Autodesk Inventor part; units mm, degrees
ref_plane "YZ Plane" through (0, 0, 0) normal (1, 0, 0) x (0, 1, 0)
ref_plane "XZ Plane" through (0, 0, 0) normal (0, 1, 0) x (-1, 0, 0)
ref_plane "XY Plane" through (0, 0, 0) normal (0, 0, 1) x (1, 0, 0)
sketch "스케치1" plane through (0, 0, 0) normal (0, 0, 1) x (1, 0, 0)
  line L0 (-71.3, 53.4) -> (-71.3, -53.4)
  line L1 (-71.3, -53.4) -> (71.3, -53.4)
  line L2 (71.3, -53.4) -> (71.3, 53.4)
  line L3 (71.3, 53.4) -> (-71.3, 53.4)
  line L4 (71.3, -53.4) -> (59.3, -53.4)
  line L5 (59.3, -53.4) -> (59.3, -47.4)
  line L6 (59.3, -47.4) -> (71.3, -47.4)
  line L7 (71.3, -47.4) -> (71.3, -53.4)
  line L8 (71.3, -53.4) -> (65.3, -53.4)
  line L9 (65.3, -53.4) -> (65.3, -41.4)
  line L10 (65.3, -41.4) -> (71.3, -41.4)
  line L11 (71.3, -41.4) -> (71.3, -53.4)
  circle A0 centre (68.3, -50.4) radius 1.35
  circle A1 centre (68.3, 50.4) radius 1.35
  circle A2 centre (-68.3, 50.4) radius 1.35
  circle A3 centre (-68.3, -50.4) radius 1.35
  circle A4 centre (68.3, -50.4) radius 1.35
  point P0 (0, 0)
  point P1 (65.3, -47.4)
  dimension "d0" = 12
  dimension "d1" = 6
  dimension "d2" = 6
  dimension "d3" = 12
  dimension "d12" = 2.7
extrude "돌출1" add sketch "스케치1" along normal blind 6 contours L5 L6 L9 L1 | L2 L6 L9 L10 | L9 L6 L2 L1
sketch "스케치2" plane through (59.3, -47.4, 0) normal (0, 1, 0) x (1, 0, 0)
  line L0 (0, 0) -> (0, -6)
  line L1 (0, -3) -> (6, -3)
  line L2 (6, 0) -> (6, -6)
  circle A0 centre (3, -3) radius 1.35
  point P0 (-59.3, 0)
  dimension "d6" = 2.7
extrude "돌출2" cut sketch "스케치2" against normal up to next
sketch "스케치3" plane through (65.3, -47.4, 0) normal (-1, 0, 0) x (0, 0, 1)
  line L0 (0, 6) -> (0, 0)
  line L1 (0, 0) -> (6, 0)
  line L2 (6, 6) -> (6, 0)
  line L3 (0, 6) -> (6, 6)
  circle A0 centre (3, 3) radius 1.35
  point P0 (0, 47.4)
  dimension "d9" = 2.7
extrude "돌출3" cut sketch "스케치3" against normal up to next contours A0
properties part number "chest_box_cap_connect"
Geometry: final body of the model. Coordinates: model frame, mm. A direction names the side the tool comes from. Round coordinates to 2 decimals unless told otherwise and drop trailing zeros. Order: outer loops, then holes, each group sorted by start corner. A loop starts at its lowest first (then second) coordinate and runs counter-clockwise, first axis right, second up. Notation, with made-up numbers: (-23, 17) - (-11, 17) arc R12 ccw to (-11, 24) - close; hole circle Ø3 at (28.5, 51.25). An arc over 180 degrees is marked (long way). Use CSV: the item, a comma, the result in double quotes. Start each with the question number.
Q1. Section query C-C (x = 62.3). Return loops of the section in (y, z).
Q2. First-contact query: pin 1 (3 mm diameter, centred on y = -45, z = 3, fed in from -X); pin 2 (2 mm diameter, centred on x = 68.3, y = -50.4, fed in from +Z); pin 3 (1.8 mm diameter, centred on x = 63, z = 3, fed in from +Y). Flat tips, straight axial feed; report the tip coordinate or a pass-through.
Q3. Section query B-B (y = -50.4). Return loops of the section in (x, z), and give its area (3 significant figures).
Q4. Section query A-A (x = 68.3). Return loops of the section in (y, z), and give its area (3 significant figures).
Q5. Mould query, pull axis Z, two halves, no side actions, for faces 1 (the face through (67, -49, 0)), 2 (the face through (65, -53.4, 3)), 3 (the face through (63.547, -50.358, 3.517)), 4 (the face through (68.26, -45.72, 2.71)). Classes: +Z half, -Z half, draft (parallel to the pull), parting line (faces both ways), or undercut.
Q6. Material intervals for line 1 along X through (y, z) = (-50.1, 3); line 2 along Y through (x, z) = (67.75, 3.7); line 3 along Y through (x, z) = (69.2, 3), sorted ascending. Write a range as from..to.
Q7. Section query D-D (z = 0.9). Return loops of the section in (x, y).
Q8. Access query for faces 5 (the face through (61, -47.4, 2)), 6 (the face through (68, -41.4, 3)). Directions: +Z, -Z, +X, -X, +Y, -Y. A direction counts if a zero-diameter tool reaches every point of the face in a straight line with its end or side. Return the directions, or none.
Result set:
1,outline,"(-53.4, 0) - (-47.4, 0) - (-47.4, 1.65) - (-53.4, 1.65) - close; (-53.4, 4.35) - (-47.4, 4.35) - (-47.4, 6) - (-53.4, 6) - close"
2,pin 1,"stops at x = 65.3"
2,pin 2,"passes through"
2,pin 3,"stops at y = -47.4"
3,outline,"(59.3, 0) - (66.95, 0) - (66.95, 6) - (59.3, 6) - close; (69.65, 0) - (71.3, 0) - (71.3, 6) - (69.65, 6) - close; hole circle Ø2.7 at (62.3, 3)"
3,area,"50.1 mm2"
4,outline,"(-53.4, 0) - (-51.75, 0) - (-51.75, 6) - (-53.4, 6) - close; (-49.05, 0) - (-41.4, 0) - (-41.4, 6) - (-49.05, 6) - close; hole circle Ø2.7 at (-44.4, 3)"
4,area,"50.1 mm2"
5,face 1,"-Z half"
5,face 2,"draft"
5,face 3,"undercut"
5,face 4,"undercut"
6,line 1,"x = 59.3..60.95, 63.65..66.98, 69.62..71.3"
6,line 2,"y = -53.4..-51.63, -49.17..-45.55, -43.25..-41.4"
6,line 3,"y = -53.4..-51.41, -49.39..-45.75, -43.05..-41.4"
7,outline,"(59.3, -53.4) - (71.3, -53.4) - (71.3, -41.4) - (65.3, -41.4) - (65.3, -47.4) - (59.3, -47.4) - close; hole circle Ø2.7 at (68.3, -50.4)"
8,face 5,"+Z, -Z, -X, +Y"
8,face 6,"+Z, -Z, +X, -X, +Y"
